from build123d import *

# Parameters (mm, degrees)
SKETCH002_R             = 15.8
SKETCH002_R_2           = 1.2
PAD002_DEPTH            = 5
POCKET_DEPTH            = 5
POLARPATTERN_COUNT      = 12
BODY002_PLACEMENT_ANGLE = 90


with BuildPart() as part:
    # Sketch002 → Pad002 (new body)
    with BuildSketch(Plane.XY):
        Circle(SKETCH002_R)
        Circle(SKETCH002_R_2, mode=Mode.SUBTRACT)
    extrude(amount=PAD002_DEPTH)

    # Sketch003 (on Face4 of Pad002) → Pocket (cut)
    with BuildSketch(Plane.XY.offset(5)):
        with BuildLine():
            ThreePointArc((-0.354655, 2.503453), (0, 2.169967), (0.354655, 2.503453))
            Line((0.354655, 2.503453), (1.071428, 14.142374))
            ThreePointArc((1.071428, 14.142374), (0, 15.281815), (-1.071428, 14.142374))
            Line((-0.354655, 2.503453), (-1.071428, 14.142374))
        make_face()
    pocket = extrude(amount=-POCKET_DEPTH, mode=Mode.SUBTRACT)

    # PolarPattern: Pocket ×12 about axis
    polarpattern_axis = Axis((0, 0, 0), (0, 0, 1))
    for i in range(1, POLARPATTERN_COUNT):
        add(pocket.rotate(polarpattern_axis, i * 360 / POLARPATTERN_COUNT), mode=Mode.SUBTRACT)


with BuildPart() as part_1:
    # Body002 placement: moved
    add(part.part.moved(Location((31, -67, 14))).rotate(Axis((31, -67, 14), (0, 1, 0)), BODY002_PLACEMENT_ANGLE))


solid = part_1.part
Model file for the job. Use its own axes, mm. A direction names the side the tool comes from. Give positions to 0.01 mm unless a question says otherwise; leave off trailing zeros. Loops run counter-clockwise (first coordinate to the right, second up) from the corner with the lowest first, then second, coordinate; pieces in that order, holes last.
Item 1: Slice it at C-C (x = 35.4). Give the number of separate pieces and of enclosed holes in the cut face, plus the area to 3 significant figures.
Check values:
separate pieces: 1
enclosed holes: 13
area: 555 mm2
Item 2: Drop flat-ended pins along their axis: P1, Ø3, axis at x = 35, z = 23, coming from the -Y side; P2, Ø12, axis at y = -59, z = 18, coming from the +X side; P3, Ø1, axis at x = 32.5, y = -60.5, coming from the -Z side. Give the stop position or say it passes through.
Check values:
P1: stops at y = -80.91
P2: stops at x = 36
P3: stops at z = -0.62
Item 3: Which spindle directions (+Z, -Z, +X, -X, +Y, -Y) get a long thin tool onto all of the face, cutting with end or side? Do faces 1 (the face through (33.53, -60.22, 18.73)), 2 (the face through (31, -70, 11)). Say none if no direction does.
Check values:
face 1: +X, -X
face 2: +Z, -Z, -X, +Y, -Y
Item 4: Mould opens along Z. For faces 3 (the face through (36, -70, 11)), 4 (the face through (33.54, -71.73, 7.22)) say: +Z half, -Z half, draft (parallel to the pull), parting line (faces both ways), or undercut.
Check values:
face 3: draft
face 4: undercut
Item 5: Drill centre lines: line 1 along Y through (x, z) = (32, 14); line 2 along Y through (x, z) = (33.6, 9.5); line 3 along Y through (x, z) = (34.4, 1.5). Where is each one in solid material? Low to high.
Check values:
line 1: y = -82.8 to -82.28, -69.17 to -68.2, -65.8 to -64.83, -51.72 to -51.2
line 2: y = -82.15 to -76.48, -73.43 to -70.22, -69.02 to -67.48, -66.52 to -64.98, -63.78 to -60.57, -57.52 to -51.85
line 3: y = -76.66 to -75.16, -73 to -67.97, -66.03 to -61, -58.84 to -57.34
Item 6: Slice it at A-A (z = 9.5). Write the cut outline in (x, y), plus the area to 3 significant figures.
Check values:
outline: (31, -82.15) - (36, -82.15) - (36, -76.48) - (31, -76.48) - close; (31, -73.43) - (36, -73.43) - (36, -70.22) - (31, -70.22) - close; (31, -69.02) - (36, -69.02) - (36, -67.48) - (31, -67.48) - close; (31, -66.52) - (36, -66.52) - (36, -64.98) - (31, -64.98) - close; (31, -63.78) - (36, -63.78) - (36, -60.57) - (31, -60.57) - close; (31, -57.52) - (36, -57.52) - (36, -51.85) - (31, -51.85) - close
area: 104 mm2
Item 7: Slice it at D-D (z = 17). Write the cut outline in (x, y), plus the area to 3 significant figures.
Check values:
outline: (31, -82.51) - (36, -82.51) - (36, -73.47) - (31, -73.47) - close; (31, -71.17) - (36, -71.17) - (36, -69.23) - (31, -69.23) - close; (31, -68.27) - (36, -68.27) - (36, -67.39) - (31, -67.39) - close; (31, -66.61) - (36, -66.61) - (36, -65.73) - (31, -65.73) - close; (31, -64.77) - (36, -64.77) - (36, -62.83) - (31, -62.83) - close; (31, -60.53) - (36, -60.53) - (36, -51.49) - (31, -51.49) - close
area: 119 mm2
Item 8: Slice it at B-B (z = 23.5). Write the cut outline in (x, y), plus the area to 3 significant figures.
Check values:
outline: (31, -79.62) - (36, -79.62) - (36, -73.53) - (31, -73.53) - close; (31, -71.51) - (36, -71.51) - (36, -67.79) - (31, -67.79) - close; (31, -66.21) - (36, -66.21) - (36, -62.49) - (31, -62.49) - close; (31, -60.47) - (36, -60.47) - (36, -54.38) - (31, -54.38) - close
area: 98.1 mm2
